For this review, use the dimensioned drawing (mm, ordinates from the lowest corner) and the shaded views. Coordinates: 2 decimals unless noted, no trailing zeros. Loops run counter-clockwise (first coordinate to the right, second up) from the corner with the lowest first, then second, coordinate; pieces in that order, holes last. Notation, with made-up numbers: M -37,-17 L 17,-17 A11 ccw 17,-9 Z; hole C -22,74.25 d1. An arc over 180 degrees is marked long. One line per item, written item: value.
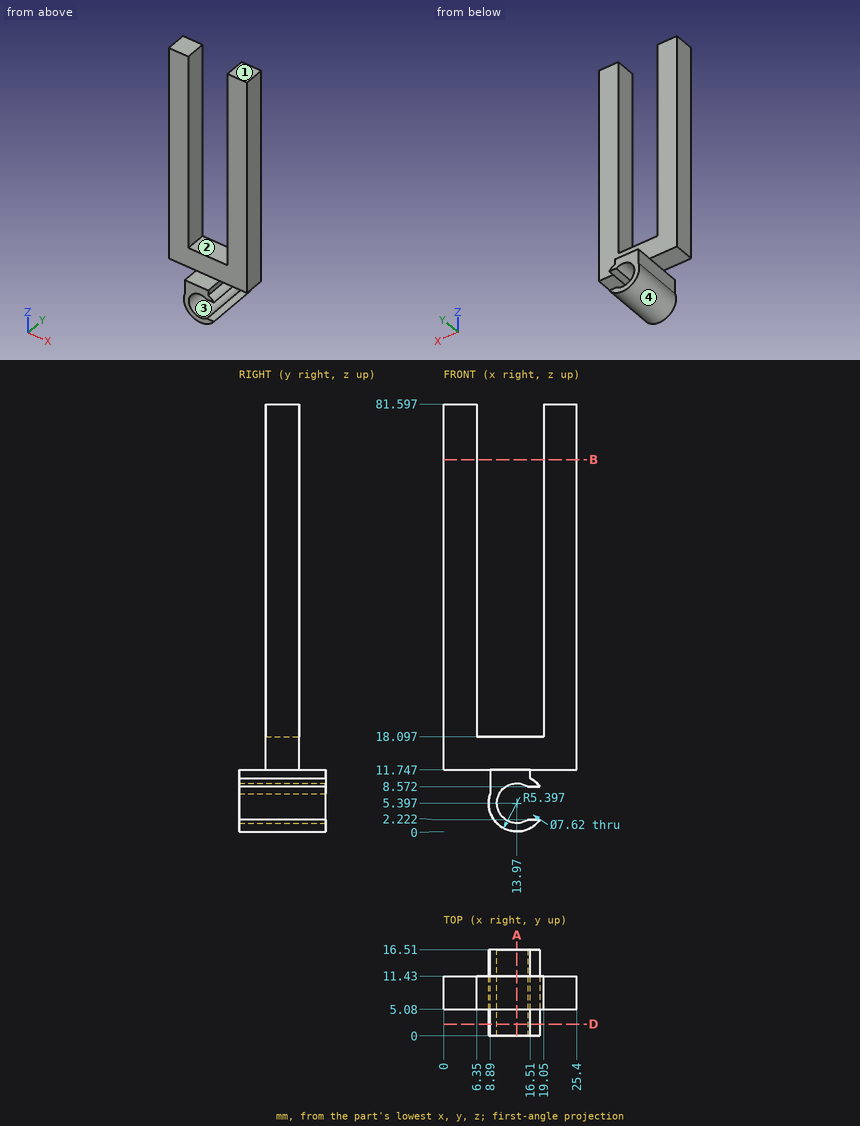
(1) Add section A-A on x = 13.97. State the section outline as (y, z) points.
Checks:
outline: M 0,0 L 16.51,0 L 16.51,1.59 L 0,1.59 Z; M 0,9.21 L 16.51,9.21 L 16.51,11.75 L 11.43,11.75 L 11.43,18.1 L 5.08,18.1 L 5.08,11.75 L 0,11.75 Z
(2) Insertion check: pin 1 Ø12 at (x, z) = (5, 64.5) entering from -Y; pin 2 Ø1.9 at (x, y) = (11, 9.5) entering from +Z; pin 3 Ø5.5 at (x, y) = (14, 1.5) entering from +Z. Each pin has a flat end and moves straight along its axis. Give the tip position at first contact, or say it passes through.
Checks:
pin 1: y = 5.08
pin 2: z = 18.1
pin 3: z = 11.75
(3) Draft analysis for pull direction X (two halves, no side actions). For the marked faces 1, 2, 3 and 4, state which applies: pulls with the +X half, pulls with the -X half, needs draft (parallel to the pull), parting line crosses it, or undercut.
Checks:
face 1: needs draft
face 2: undercut
face 3: undercut
face 4: parting line crosses it
(4) To check wall thickness, follow L1, parallel to X at y = 8.5, z = 63.5; L2, parallel to Z at x = 13.97, y = 7; L3, parallel to Z at x = 13.97, y = 4. State the ranges of each line that lie inside material, in increasing order. Write a range as [from, to].
Checks:
L1: [0, 6.35], [19.05, 25.4]
L2: [0, 1.59], [9.21, 18.1]
L3: [0, 1.59], [9.21, 11.75]
(5) Add section D-D on y = 2.25. State the section outline as (x, z) points (1 decimal).
Checks:
outline: M 8.9,7.2 A5.4 ccw 18.3,2.2 L 16.1,2.2 A3.8 cw long 16.1,8.6 L 18.3,8.6 A5.4 ccw 16.5,10.2 L 16.5,11.7 L 8.9,11.7 Z
(6) Add section B-B on z = 71. State the section outline as (x, y) points.
Checks:
outline: M 0,5.08 L 6.35,5.08 L 6.35,11.43 L 0,11.43 Z; M 19.05,5.08 L 25.4,5.08 L 25.4,11.43 L 19.05,11.43 Z
